Autodesk Inventor part; units mm, degrees
ref_plane "YZ Plane" through (0, 0, 0) normal (1, 0, 0) x (0, 1, 0)
ref_plane "XZ Plane" through (0, 0, 0) normal (0, 1, 0) x (-1, 0, 0)
ref_plane "XY Plane" through (0, 0, 0) normal (0, 0, 1) x (1, 0, 0)
sketch "Sketch5" plane through (0, 0, 0) normal (1, 0, 0) x (0, 1, 0)
  line L0 (76, -76) -> (-76, -76)
  line L1 (-76, -76) -> (-76, 76)
  line L2 (-76, 76) -> (76, 76)
  line L3 (76, 76) -> (76, -76)
  line L4 (76, -76) -> (-76, 76) construction
  line L5 (-76, -76) -> (76, 76) construction
  point P0 (0, 0)
  dimension "d31" = 152
  dimension "d32" = 152
extrude "Extrusion2" add sketch "Sketch5" along normal blind 10
sketch "Sketch6" plane through (10, 0, 0) normal (1, 0, 0) x (0, 0, -1)
  line L0 (76, -76) -> (76, 76)
  line L1 (76, 76) -> (-76, 76)
  point P0 (0, 0)
  point P1 (50.6, 50.6)
  dimension "d42" = 25.4
  dimension "d43" = 25.4
hole "Hole4" at (10, 50.6, -50.6) direction (-1, 0, 0) diameter 14.3 end through all
sketch "Sketch7" plane through (10, 0, 0) normal (1, 0, 0) x (0, 0, -1)
  circle A0 centre (50.6, 50.6) radius 7.15
  line L0 (76, 76) -> (-76, 76)
  point P0 (0, 0)
  point P1 (-51, 50.6)
  dimension "d51" = 101.6
  dimension "d52" = 25.4
hole "Hole5" at (10, 50.6, 51) direction (-1, 0, 0) diameter 14.3 end through all
sketch "Sketch8" plane through (10, 0, 0) normal (1, 0, 0) x (0, 0, -1)
  line L0 (76, -76) -> (76, 76)
  circle A0 centre (50.6, 50.6) radius 7.15
  point P0 (0, 0)
  point P1 (50.6, -51)
  dimension "d60" = 25.4
  dimension "d61" = 101.6
hole "Hole6" at (10, -51, -50.6) direction (-1, 0, 0) diameter 14.3 end through all
sketch "Sketch9" plane through (10, 0, 0) normal (1, 0, 0) x (0, 0, -1)
  circle A0 centre (-51, 50.6) radius 7.15
  circle A1 centre (50.6, -51) radius 7.15
  point P0 (0, 0)
  point P1 (-51, -51)
  dimension "d69" = 101.6
  dimension "d70" = 101.6
hole "Hole7" at (10, -51, 51) direction (-1, 0, 0) diameter 14.3 end through all
sketch "Sketch10" plane through (10, 0, 0) normal (1, 0, 0) x (0, 0, -1)
  line L0 (76, 76) -> (-76, 76)
  line L1 (76, -76) -> (76, 76)
  point P0 (0, 0)
  point P1 (19.05, 63.5)
  dimension "d93" = 12.5
  dimension "d103" = 56.95
hole "Hole8" at (10, 63.5, -19.05) direction (-1, 0, 0) diameter 6.8 end through all
sketch "Sketch11" plane through (10, 0, 0) normal (1, 0, 0) x (0, 0, -1)
  circle A0 centre (19.05, 63.5) radius 3.4
  point P0 (0, 0)
  point P1 (-19.05, 63.5)
  dimension "d85" = 38.1
  dimension "d86" = 0
hole "Hole9" at (10, 63.5, 19.05) direction (-1, 0, 0) diameter 6.8 end through all
pattern_linear "Rectangular Pattern1" count 6 spacing 25.4 along (0, -1, 0) of "Hole8"
pattern_linear "Rectangular Pattern2" count 6 spacing 25.4 along (0, -1, 0) of "Hole9"
sketch "Sketch12" plane through (10, 0, 0) normal (1, 0, 0) x (0, 0, -1)
  line L0 (76, -76) -> (76, 76)
  line L1 (-76, -76) -> (76, -76)
  point P0 (0, 0)
  point P1 (0, 0)
  dimension "d101" = 76
  dimension "d102" = 76
hole "Hole10" at (10, 0, 0) direction (-1, 0, 0) diameter 5.2 end through all
properties part number "base_plate"
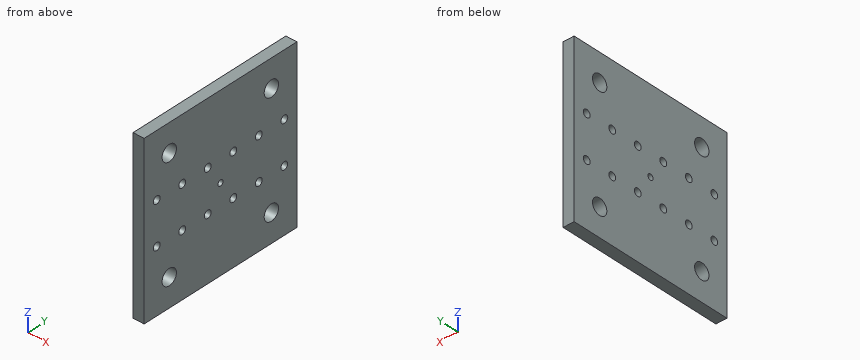
The model under review builds one solid part; all positions refer to its coordinate system, in mm. Round coordinates to 2 decimals unless told otherwise and drop trailing zeros. Order: outer loops, then holes, each group sorted by start corner. A loop starts at its lowest first (then second) coordinate and runs counter-clockwise, first axis right, second up. Notation, with made-up numbers: (58.5, -14.5) -> (104.5, -14.5) arc R32 cw to (104.5, 14.5) -> close; hole circle Ø6 at (33, 49). An arc over 180 degrees is marked (long way). Use a Markdown table: item, result.
Q1. For line 1 (Z direction, x = 5, y = 50.6); line 2 (Z direction, x = 2.75, y = 12.7); line 3 (Y direction, x = 2.75, z = 0), list the stretches that pass through material, from the lowest coordinate up.
Values:
| item | result |
|---|---|
| line 1 | z = -76 to -57.75, -43.45 to 43.85, 58.15 to 76 |
| line 2 | z = -76 to -22.45, -15.65 to 15.65, 22.45 to 76 |
| line 3 | y = -76 to -2.6, 2.6 to 76 |
Q2. We need section A-A on z = 19.05. Write out the cut boundary in (x, y), then the cut area to 3 significant figures.
Values:
| item | result |
|---|---|
| outline | (0, -76) -> (10, -76) -> (10, -66.9) -> (0, -66.9) -> close; (0, -60.1) -> (10, -60.1) -> (10, -41.5) -> (0, -41.5) -> close; (0, -34.7) -> (10, -34.7) -> (10, -16.1) -> (0, -16.1) -> close; (0, -9.3) -> (10, -9.3) -> (10, 9.3) -> (0, 9.3) -> close; (0, 16.1) -> (10, 16.1) -> (10, 34.7) -> (0, 34.7) -> close; (0, 41.5) -> (10, 41.5) -> (10, 60.1) -> (0, 60.1) -> close; (0, 66.9) -> (10, 66.9) -> (10, 76) -> (0, 76) -> close |
| area | 1,110 mm^2 |
Q3. Clearance check with a flat-ended pin moving along its axis: P1, Ø4, axis at y = 12.7, z = 19.05, coming from the -X side. State where the tip first meets the part, or that it passes through.
Values:
| item | result |
|---|---|
| P1 | passes through |
Q4. We need section B-B on y = -63.5. Write out the cut boundary in (x, z), then the cut area to 3 significant figures.
Values:
| item | result |
|---|---|
| outline | (0, -76) -> (10, -76) -> (10, -22.45) -> (0, -22.45) -> close; (0, -15.65) -> (10, -15.65) -> (10, 15.65) -> (0, 15.65) -> close; (0, 22.45) -> (10, 22.45) -> (10, 76) -> (0, 76) -> close |
| area | 1,380 mm^2 |
Q5. We need section D-D on x = 5. State how many separate pieces and enclosed holes the cut face has, then the cut area to 3 significant figures.
Values:
| item | result |
|---|---|
| separate pieces | 1 |
| enclosed holes | 17 |
| area | 22,000 mm^2 |
Q6. We need section C-C on z = 51. Write out the cut boundary in (x, y).
Values:
| item | result |
|---|---|
| outline | (0, -76) -> (10, -76) -> (10, -58.15) -> (0, -58.15) -> close; (0, -43.85) -> (10, -43.85) -> (10, 43.45) -> (0, 43.45) -> close; (0, 57.75) -> (10, 57.75) -> (10, 76) -> (0, 76) -> close |
